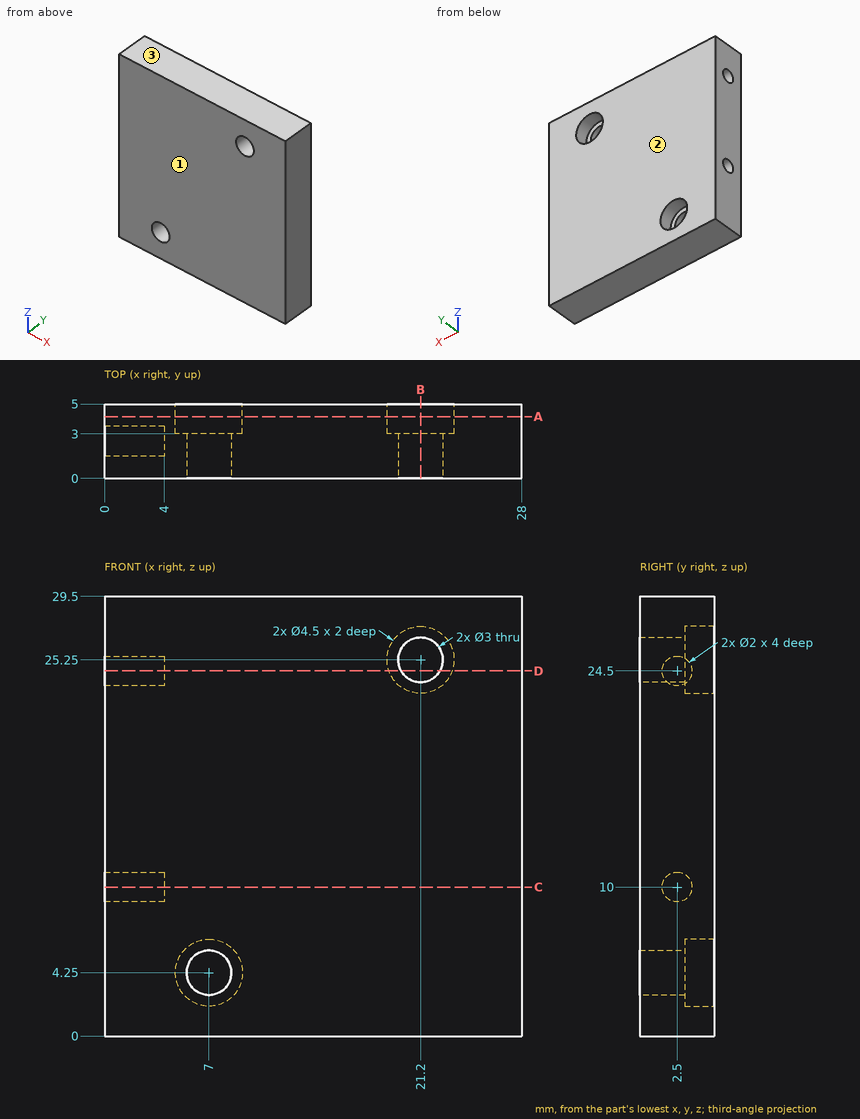
Can you work these out from the drawing? Everything is in mm from the part's minimum corner. Give positions to 0.01 mm unless a question says otherwise; leave off trailing zeros. Loops run counter-clockwise (first coordinate to the right, second up) from the corner with the lowest first, then second, coordinate; pieces in that order, holes last. Notation, with made-up numbers: (26, 24.5) - (73, 24.5) arc R20 cw to (73, 59.5) - close; hole circle Ø4 at (61, -27). An arc over 180 degrees is marked (long way). Use one line per item in the form item = value.
1. I want a section at B-B (x = 21.2). Please give me the cut outline in (y, z), and give its area (4 significant figures).
Response values:
outline = (0, 0) - (5, 0) - (5, 23) - (3, 23) - (3, 23.75) - (0, 23.75) - close; (0, 26.75) - (3, 26.75) - (3, 27.5) - (5, 27.5) - (5, 29.5) - (0, 29.5) - close
area = 129.5 mm²
2. Thinking about a two-plate mould opening in Y: for the marked faces 1, 2 and 3, which applies, released by +Y, released by -Y, zero draft, split by the parting line, or undercut?
Response values:
face_1 = released by -Y
face_2 = released by +Y
face_3 = zero draft
3. I'm going to push flat-ended pins straight in: pin 1 Ø1.3 at (x, z) = (6.5, 4.5) entering from +Y; pin 2 Ø2 at (y, z) = (2.5, 24) entering from -X; pin 3 Ø4 at (x, z) = (21.2, 25.25) entering from +Y. Where does each tip first touch, or does it pass through?
Response values:
pin_1 = through
pin_2 = 0
pin_3 = 3
4. I want a section at D-D (z = 24.5). Please give me the cut outline in (x, y), and give its area (3 significant figures).
Response values:
outline = (0, 0) - (19.9, 0) - (19.9, 3) - (19.08, 3) - (19.08, 5) - (0, 5) - (0, 3.5) - (4, 3.5) - (4, 1.5) - (0, 1.5) - close; (22.5, 0) - (28, 0) - (28, 5) - (23.32, 5) - (23.32, 3) - (22.5, 3) - close
area = 116 mm²
5. I want a section at A-A (y = 4.15). Please give me the cut outline in (x, z), and give its area (3 significant figures).
Response values:
outline = (0, 0) - (28, 0) - (28, 29.5) - (0, 29.5) - close; hole circle Ø4.5 at (7, 4.25); hole circle Ø4.5 at (21.2, 25.25)
area = 794 mm²
6. I need wall thicknesses on probe 1 along X at (y, z) = (1.85, 4.25); probe 2 along Y at (x, z) = (2.9, 10); probe 3 along Z at (x, y) = (21.2, 1). Which ranges of each line are inside material? Lowest first, please.
Response values:
probe_1 = 0 to 5.5, 8.5 to 28
probe_2 = 0 to 1.5, 3.5 to 5
probe_3 = 0 to 23.75, 26.75 to 29.5
7. I want a section at C-C (z = 10). Please give me the cut outline in (x, y).
Response values:
outline = (0, 0) - (28, 0) - (28, 5) - (0, 5) - (0, 3.5) - (4, 3.5) - (4, 1.5) - (0, 1.5) - close
